from build123d import *

# Parameters (mm, degrees)
SKETCH1_W           = 60
SKETCH1_H           = 65
BOSS_EXTRUDE1_DEPTH = 25
CUT_EXTRUDE1_DEPTH  = 60
SKETCH4_R           = 5
CUT_EXTRUDE2_DEPTH  = 51
FILLET1_R           = 10
SCALE1_SCALE        = 0.3


with BuildPart() as part:
    # Sketch1 → Boss-Extrude1 (new body, symmetric)
    with BuildSketch(Plane.XY):
        with Locations((-3.578258959, -17.200317296)):
            Rectangle(SKETCH1_W, SKETCH1_H)
    extrude(amount=BOSS_EXTRUDE1_DEPTH, both=True)

    # Sketch3 → Cut-Extrude1 (cut)
    with BuildSketch(Plane(origin=(26.421741041, 0, 0), x_dir=(0, 0, -1), z_dir=(1, 0, 0))):
        Polygon((-15, 5.299682704), (15, 5.299682704), (6, 15.299682704), (-6, 15.299682704), align=None)
    extrude(amount=-CUT_EXTRUDE1_DEPTH, mode=Mode.SUBTRACT)

    # Sketch4 → Cut-Extrude2 (cut, through all)
    with BuildSketch(Plane.XY.offset(25)):
        with Locations((16.421741041, -39.700317296)):
            Circle(SKETCH4_R)
        with Locations((-23.578258959, -39.700317296)):
            Circle(SKETCH4_R)
    extrude(amount=-CUT_EXTRUDE2_DEPTH, mode=Mode.SUBTRACT)

    # Fillet1
    fillet1_edges = [part.edges().sort_by_distance(p)[0] for p in [
        (26.421741041, -49.700317296, 0),
        (-33.578258959, -49.700317296, 0),
    ]]
    fillet(fillet1_edges, radius=FILLET1_R)


with BuildPart() as part_1:
    # Scale1: scaled about (-3.578258959, -17.756195099, 0)
    add(part.part.scale(SCALE1_SCALE).moved(Location((-2.504781271, -12.429336569, 0))))


solid = part_1.part
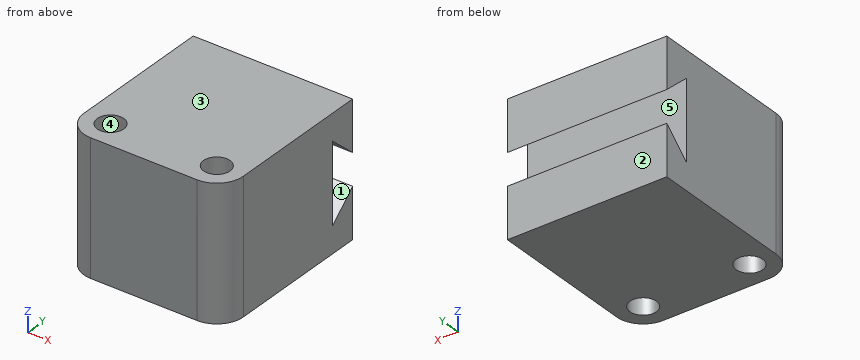
Geometry: final body of the model. Coordinates: model frame, mm. Face numbers are marked on the shaded views. A direction names the side the tool comes from. Give positions to 0.01 mm unless a question says otherwise; leave off trailing zeros. Write each loop counter-clockwise with the first axis right and the second up, starting at its lowest first coordinate (ties: lowest second). Pieces come first, ordered by that corner, then holes.
(1) Cut plane C-C, the plane z = 3.75. Return loops of the section in (x, y).
(2) Cut plane B-B, the plane y = -10.5. Return loops of the section in (x, z).
(3) First-contact query: P1, Ø5, axis at x = 2.42, y = -24.34, coming from the -Z side. Flat tip, straight axial feed; report the tip coordinate or a pass-through.
(4) Mould query, pull axis Z, two halves, no side actions, for the marked faces 3, 4 and 5. Classes: released by +Z, released by -Z, zero draft, split by the parting line, or undercut.
(5) Cut plane D-D, the plane x = -10.5. Return loops of the section in (y, z).
(6) Cut plane A-A, the plane z = -1.5. Return loops of the section in (x, y).
(7) Access query for the marked faces 1 and 2. Directions: +Z, -Z, +X, -X, +Y, -Y. A direction counts if a zero-diameter tool reaches every point of the face in a straight line with its end or side. Return the directions, or none.
(8) Ray query, line 1 (X direction, y = -25, z = -3.5); line 2 (Y direction, x = 2.5, z = 4.25); line 3 (X direction, y = -24, z = -2.5). Return the intervals inside material, ascending.
Values follow:
1. outline: (-12.58, -24.34) arc R3 ccw to (-9.58, -27.34) - (2.42, -27.34) arc R3 ccw to (5.42, -24.34) - (5.42, -10.84) - (-12.58, -10.84) - close; (-12.58, -10.01) - (5.42, -10.01) - (5.42, -7.84) - (-12.58, -7.84) - close; hole circle Ø3 at (-9.58, -24.34); hole circle Ø3 at (2.42, -24.34)
2. outline: (-12.58, -7.5) - (5.42, -7.5) - (5.42, -4.19) - (-12.58, -4.19) - close; (-12.58, 4.19) - (5.42, 4.19) - (5.42, 7.5) - (-12.58, 7.5) - close
3. P1: stops at z = -7.5
4. face 3: released by +Z
4. face 4: zero draft
4. face 5: undercut
5. outline: (-27.19, -7.5) - (-25.52, -7.5) - (-25.52, 7.5) - (-27.19, 7.5) - close; (-23.16, -7.5) - (-7.84, -7.5) - (-7.84, -1.8) - (-10.84, -4.5) - (-10.84, 4.5) - (-7.84, 1.8) - (-7.84, 7.5) - (-23.16, 7.5) - close
6. outline: (-12.58, -24.34) arc R3 ccw to (-9.58, -27.34) - (2.42, -27.34) arc R3 ccw to (5.42, -24.34) - (5.42, -10.84) - (-12.58, -10.84) - close; hole circle Ø3 at (-9.58, -24.34); hole circle Ø3 at (2.42, -24.34)
7. face 1: +X, -X
7. face 2: +Z, -Z, +X, -X, +Y
8. line 1: x = -12.5 to -10.92, -8.23 to 1.08, 3.77 to 5.35
8. line 2: y = -27.34 to -25.84, -22.84 to -10.84, -10.56 to -7.84
8. line 3: x = -12.58 to -11.04, -8.12 to 0.96, 3.88 to 5.42
